Autodesk Inventor part; units mm, degrees
ref_plane "Płaszczyzna konstrukcyjna1" through (-138.5, 0, -1) normal (0, 0, 1) x (1, 0, 0)
ref_plane "YZ Plane" through (0, 0, 0) normal (1, 0, 0) x (0, 1, 0)
ref_plane "XZ Plane" through (0, 0, 0) normal (0, 1, 0) x (-1, 0, 0)
sketch "Szkic1" plane through (0, 0, 0) normal (0, 1, 0) x (-1, 0, 0)
  line L0 (0, 0) -> (150, 0)
  line L1 (150, 0) -> (150, -5)
  line L2 (150, -5) -> (0, -5)
  line L3 (0, -5) -> (0, 0)
  dimension "d0" = 150
  dimension "d1" = 5
extrude "Wyciągnięcie proste1" add sketch "Szkic1" along normal blind 20
sketch "Szkic2" plane through (0, 0, -5) normal (0, 0, -1) x (-1, 0, 0)
  line L0 (0, 0) -> (0, 20)
  circle A0 centre (0, 10) radius 2.95
  line L1 (0, 20) -> (-2, 20)
  line L2 (0, 0) -> (-2, 0)
  arc A1 (-2, 20) -> (-2, 0) centre (9.1803, 10) ccw
  line L3 (0, 10) -> (150, 10)
  line L4 (150, 10) -> (138.5, 10)
  line L5 (138.5, 10) -> (170.9, 10)
  line L6 (150, 0) -> (150, 20)
  line L7 (138.5, 10) -> (170.9, 10) construction
  line L8 (138.5, 10) -> (170.9, 10)
  line L9 (170.9, 10) -> (170.9, 16.16)
  line L10 (170.9, 16.16) -> (138.5, 16.16)
  line L11 (138.5, 16.16) -> (138.5, 10)
  line L12 (138.5, 10) -> (170.9, 10)
  line L13 (170.9, 10) -> (170.9, 3.84)
  line L14 (170.9, 3.84) -> (138.5, 3.84)
  line L15 (138.5, 3.84) -> (138.5, 10)
  line L16 (0, 0) -> (150, 0)
  line L17 (0, 20) -> (150, 20)
  arc A2 (138.5, 0) -> (138.5, 20) centre (154.9429, 10) ccw
  point P0 (150, 3.84)
  point P1 (150, 16.16)
  point P2 (0, 7.05)
  point P3 (0, 12.95)
  dimension "d4" = 5.9
  dimension "d5" = 2
  dimension "d6" = 2
  dimension "d7" = 15
  dimension "d8" = 150
  dimension "d9" = 11.5
  dimension "d10" = 32.4
  dimension "d11" = 0
  dimension "d12" = 6.16
  dimension "d13" = 6.16
extrude "Wyciągnięcie proste2" add sketch "Szkic2" against normal blind 5 contours L2 A1 L1 L0 A0 | L16 L6 L14 L13 L9 L10 L17 A2
sketch "Szkic3" plane through (2, 20, -5) normal (0, 0, -1) x (-1, 0, 0)
  arc A0 (2, -7.05) -> (2, -12.95) centre (2, -10) ccw
  circle A1 centre (2, -10) radius 2.95
  line L0 (152, -16.16) -> (152, -3.84)
  line L1 (152, -16.16) -> (150.5, -16.16)
  line L2 (150.5, -16.16) -> (150.5, -3.84)
  line L3 (150.5, -3.84) -> (152, -3.84)
  line L4 (140.5, -16.16) -> (10.5, -16.16)
  line L5 (10.5, -16.16) -> (10.5, -3.84)
  line L6 (10.5, -3.84) -> (140.5, -3.84)
  line L7 (140.5, -3.84) -> (140.5, -16.16)
  line L8 (150.5, -16.16) -> (150.3, -16.16)
  line L9 (150.3, -16.16) -> (150.3, -3.84)
  line L10 (150.3, -3.84) -> (150.5, -3.84)
  line L11 (152, -16.16) -> (140.5, -16.16)
  line L12 (140.5, -16.16) -> (140.5, -3.84)
  line L13 (140.5, -3.84) -> (152, -3.84)
  line L14 (152, -3.84) -> (152, -16.16)
  point P0 (2, -20)
  dimension "d16" = 1.5
  dimension "d17" = 130
  dimension "d18" = 12.32
  dimension "d21" = 0.2
  dimension "d24" = 11.5
extrude "Wyciągnięcie proste3" cut sketch "Szkic3" against normal through all
sketch "Szkic5" plane through (2, 20, -5) normal (0, 0, -1) x (-1, 0, 0)
  circle A0 centre (2, -10) radius 2.95
  line L0 (2, -10) -> (152, -10)
  line L1 (2, -10) -> (152, -10) construction
  circle A1 centre (152, -10) radius 5.0551
  line L2 (152, -10) -> (145.8, -10)
  line L3 (145.8, -10) -> (145.8, -3.84)
  line L4 (10.5, -3.84) -> (172.9, -3.84)
  line L5 (145.8, -3.84) -> (140.8, -3.84)
  line L6 (140.8, -3.84) -> (140.8, -16.16)
  line L7 (172.9, -16.16) -> (10.5, -16.16)
  line L8 (145.8, -10) -> (145.8, -16.16)
  line L9 (145.8, -16.16) -> (140.8, -16.16)
  line L10 (10.5, -16.16) -> (10.5, -3.84)
  line L11 (10.5, -16.16) -> (44.3489, -3.84)
  line L12 (10.5, -16.16) -> (46.5213, -16.16) construction
  line L13 (44.3489, -3.84) -> (54.3489, -3.84)
  line L14 (10.5, -16.16) -> (20.5, -16.16)
  line L15 (20.5, -16.16) -> (54.3489, -3.84)
  line L16 (20.5, -16.16) -> (30.5, -16.16)
  line L17 (54.3489, -3.84) -> (64.3489, -3.84)
  line L18 (64.3489, -3.84) -> (30.5, -16.16)
  line L19 (44.3489, -3.84) -> (34.3489, -3.84)
  line L20 (10.5, -16.16) -> (0.5, -16.16)
  line L21 (0.5, -16.16) -> (34.3489, -3.84)
  line L22 (40.5, -16.16) -> (74.3489, -3.84)
  line L23 (50.5, -16.16) -> (84.3489, -3.84)
  line L24 (94.3489, -3.84) -> (60.5, -16.16)
  line L25 (30.5, -16.16) -> (64.3489, -3.84)
  line L26 (70.5, -16.16) -> (104.3489, -3.84)
  line L27 (80.5, -16.16) -> (114.3489, -3.84)
  line L28 (124.3489, -3.84) -> (90.5, -16.16)
  line L29 (60.5, -16.16) -> (94.3489, -3.84)
  line L30 (100.5, -16.16) -> (134.3489, -3.84)
  line L31 (110.5, -16.16) -> (144.3489, -3.84)
  line L32 (90.5, -16.16) -> (124.3489, -3.84)
  point P0 (2, -20)
  point P1 (10.5, -12.5203)
  point P2 (60.5, -16.16)
  point P3 (140.8, -5.1317)
  dimension "d25" = 150
  dimension "d26" = 0
  dimension "d27" = 6.2
  dimension "d28" = 5
  dimension "d29" = 20
  dimension "d30" = 10
  dimension "d31" = 10
  dimension "d32" = 10
  dimension "d33" = 10
  dimension "d34" = 10
  dimension "d35" = 10
  dimension "d36" = 10
  dimension "d37" = 10
  dimension "d38" = 10
  dimension "d39" = 10
  dimension "d40" = 10
  dimension "d41" = 10
  dimension "d42" = 10
  dimension "d43" = 10
  dimension "d44" = 10
  dimension "d45" = 10
  dimension "d46" = 10
  dimension "d47" = 10
  dimension "d48" = 10
  dimension "d49" = 10
  dimension "d52" = 10
  dimension "d53" = 10
extrude "Wyciągnięcie proste4" add sketch "Szkic5" against normal blind 5 contours L21 L4 L11 L0 | L0 L11 L10 L21 | L15 L4 L18 L0 | L0 L18 L7 L15 | L22 L4 L23 L0 | L0 L23 L7 L22 | L24 L4 L26 L0 | L0 L26 L7 L24 | L27 L4 L28 L0 | L0 L28 L7 L27 | L30 L4 L6 L31 L0 | L0 L31 L7 L30 | L6 L31 L4 L3 L0 | L0 L8 L7 L6 | L6 L4 L31
sketch "Szkic6" plane through (-138.5, 0, 0) normal (0, 0, 1) x (1, 0, 0)
  circle A0 centre (138.5, 10) radius 2.95
  circle A1 centre (138.5, 10) radius 2.85
  circle A2 centre (138.5, 10) radius 2.95
  point P0 (138.5, 0)
  dimension "d56" = 5.7
extrude "Wyciągnięcie proste5" add sketch "Szkic6" against normal blind 5
ref_plane "Płaszczyzna konstrukcyjna1" through (-138.5, 0, -1) normal (0, 0, 1) x (1, 0, 0)
sketch "Szkic7" plane through (-138.5, 0, -1) normal (0, 0, 1) x (1, 0, 0)
  circle A0 centre (138.5, 10) radius 2.85
  circle A1 centre (138.5, 10) radius 1.25
  circle A2 centre (138.5, 10) radius 2.85
  point P0 (138.5, 0)
  dimension "d60" = 2.5
extrude "Wyciągnięcie proste6" add sketch "Szkic7" against normal blind 2
sketch "Szkic8" plane through (-138.5, 0, 0) normal (0, 0, 1) x (1, 0, 0)
  point P0 (138.5, 0)
sketch "Szkic9" plane through (-138.5, 0, 0) normal (0, 0, 1) x (1, 0, 0)
  circle A0 centre (138.5, 10) radius 1.25
  line L0 (138.5, 10) -> (-11.5, 10)
  line L1 (138.5, 10) -> (288.5, 10) construction
  circle A1 centre (-11.5, 10) radius 8.15
  point P0 (138.5, 0)
  dimension "d63" = 150
  dimension "d64" = 180
  dimension "d65" = 16.3
extrude "Wyciągnięcie proste7" cut sketch "Szkic9" against normal through all contours A1
sketch "Szkic10" plane through (-138.5, 0, 0) normal (0, 0, 1) x (1, 0, 0)
  arc A0 (-5.3, 4.7102) -> (-5.3, 15.2898) centre (-11.5, 10) ccw
  circle A1 centre (-11.5, 10) radius 8.15
  line L0 (-32.5164, 20) -> (-2.9538, 20)
  line L1 (-2.9538, 20) -> (-2.9538, 1.85)
  line L2 (-2.9538, 1.85) -> (-32.5164, 1.85)
  line L3 (-32.5164, 1.85) -> (-32.5164, 20)
  point P0 (138.5, 0)
  point P1 (-11.5, 1.85)
  point P2 (-5.3, 15.2898)
extrude "Wyciągnięcie proste8" add sketch "Szkic10" against normal blind 5
sketch "Szkic11" plane through (2, 20, -5) normal (0, 0, -1) x (-1, 0, 0)
  circle A0 centre (152, -10) radius 8.15
  circle A1 centre (152, -10) radius 8.15
  circle A2 centre (152, -10) radius 10
  point P0 (2, -20)
  dimension "d70" = 20
extrude "Wyciągnięcie proste9" add sketch "Szkic11" along normal blind 3
sketch "Szkic12" plane through (-138.5, 0, 0) normal (0, 0, 1) x (1, 0, 0)
  line L0 (135.65, 12.85) -> (141.4166, 12.85)
  line L1 (141.4166, 12.85) -> (141.4166, 7.15)
  line L2 (141.4166, 7.15) -> (135.65, 7.15)
  line L3 (135.65, 7.15) -> (135.65, 12.85)
  circle A0 centre (138.5, 10) radius 2.85
  line L4 (141.35, 10) -> (141.35, 7.15)
  line L5 (141.35, 10) -> (141.35, 12.85)
  point P0 (138.5, 0)
extrude "Wyciągnięcie proste10" cut sketch "Szkic12" against normal blind 0.5 contours A0
chamfer "Faza1" distance 1 angle 45 1 edges at (-2.85, 10, 0)
sketch "Szkic13" plane through (2, 20, -5) normal (0, 0, -1) x (-1, 0, 0)
  circle A0 centre (2, -10) radius 2.85
  circle A1 centre (2, -10) radius 2.85
  circle A2 centre (2, -10) radius 2.825
  point P0 (2, -20)
  dimension "d78" = 5.65
extrude "Wyciągnięcie proste11" add sketch "Szkic13" against normal blind 4
properties part number "arm_v3_backup"
Can you work these out from the model? Positions are in its coordinate system, mm. A direction names the side the tool comes from. Give positions to 0.01 mm unless a question says otherwise; leave off trailing zeros. Loops run counter-clockwise (first coordinate to the right, second up) from the corner with the lowest first, then second, coordinate; pieces in that order, holes last. Notation, with made-up numbers: (-32, -6.75) - (-22, -6.75) arc R30 ccw to (-22, 19.25) - close; hole circle Ø10 at (11.25, -16.5). An arc over 180 degrees is marked (long way). Answer as a JSON object with one key per item and string values.
Q1. If we mould it in two halves opening along Y, with no side actions, what happens to faces 1 (the flat face through (-67, 20, -2)), 2 (the flat face through (-107, 16.16, -3)), 3 (the flat face through (-67, 0, -2))? For each: pulls with the +Y half, pulls with the -Y half, needs draft (parallel to the pull), parting line crosses it, or undercut.
Geometry says:
{"face 1": "pulls with the +Y half", "face 2": "undercut", "face 3": "pulls with the -Y half"}
Q2. Imagine slicing it at B-B on x = -150. Write out the boundary of the cut face in (y, z).
Geometry says:
{"outline": "(-8.6, -5) - (0, -5) - (0, -8) - (1.85, -8) - (1.85, 0) - (-8.6, 0) - close; (18.15, -8) - (20, -8) - (20, -5) - (28.6, -5) - (28.6, 0) - (18.15, 0) - close"}
Q3. Will these pins go through, and if not, where does the flat tip stop? P1, Ø2.5, axis at x = -46, z = -3.5, coming from the -Y side; P2, Ø4.5, axis at x = 0, y = 10, coming from the +Z side; P3, Ø1.5, axis at y = 12, z = -1.5, coming from the -X side.
Geometry says:
{"P1": "y = 0", "P2": "z = -1", "P3": "x = -174.15"}
Q4. Imagine slicing it at C-C on x = -11. Write out the boundary of the cut face in (y, z), plus the area to 3 significant figures.
Geometry says:
{"outline": "(0, -5) - (3.84, -5) - (3.84, 0) - (0, 0) - close; (4.75, -5) - (8.39, -5) - (8.39, 0) - (4.75, 0) - close; (16.16, -5) - (20, -5) - (20, 0) - (16.16, 0) - close", "area": "56.6 mm²"}
Q5. Imagine slicing it at A-A on x = -76.5. Write out the boundary of the cut face in (y, z), plus the area to 3 significant figures.
Geometry says:
{"outline": "(0, -5) - (3.84, -5) - (3.84, 0) - (0, 0) - close; (6.75, -5) - (10.39, -5) - (10.39, 0) - (6.75, 0) - close; (14.03, -5) - (20, -5) - (20, 0) - (14.03, 0) - close", "area": "67.2 mm²"}
Q6. If I drill on L1, parallel to Y at x = 0, z = -1.95; L2, parallel to Y at x = -87.5, z = -4.75; L3, parallel to Y at x = -90, z = -4.75, over which ranges is the centre line in solid material (lowest first)?
Geometry says:
{"L1": "0 to 8.75, 11.25 to 20", "L2": "0 to 7.12, 10.76 to 14.4, 16.16 to 20", "L3": "0 to 3.84, 4.39 to 8.03, 11.67 to 15.31, 16.16 to 20"}
Q7. Which directions (+Z, -Z, +X, -X, +Y, -Y) give clear straight access to the entire face, cutting with the end or side of a thin tool? Please do faces 4 (the flat face through (1, 9, -3)), 5 (the flat face through (-95.188, 9.914, -2.535)), 6 (the flat face through (-146.2, 2.6, -8)).
Geometry says:
{"face 4": "-Z", "face 5": "+Z, -Z", "face 6": "-Z, +X, -X, +Y, -Y"}
Q8. Imagine slicing it at D-D on y = -3. Write out the boundary of the cut face in (x, z), plus the area to 3 significant figures.
Geometry says:
{"outline": "(-169.13, -5) - (-140.75, -5) - (-140.75, 0) - (-169.13, 0) - close", "area": "142 mm²"}
